from build123d import *

# Parameters (mm, degrees)
SKETCH1_R           = 1.0287
SKETCH1_R_2         = 1.47
BOSS_EXTRUDE1_DEPTH = 1.5875


with BuildPart() as part:
    # Sketch1 → Boss-Extrude1 (new body, symmetric)
    with BuildSketch(Plane.XY):
        Polygon((-12.5, 50), (-56.825, 50), (-56.825, 12.5), (-60, 12.5), (-60, -12.5), (-56.825, -12.5), (-56.825, -50), (-12.5, -50), (-12.5, -46.825), (-1.47, -46.825), (-1.47, -43.125), (-3.25, -43.125), (-3.25, -40.525), (-1.47, -40.525), (-1.47, -36.825), (1.47, -36.825), (1.47, -40.525), (3.25, -40.525), (3.25, -43.125), (1.47, -43.125), (1.47, -46.825), (12.5, -46.825), (12.5, -50), (56.825, -50), (56.825, -12.5), (60, -12.5), (60, 12.5), (56.825, 12.5), (56.825, 50), (12.5, 50), (12.5, 46.825), (1.47, 46.825), (1.47, 43.125), (3.25, 43.125), (3.25, 40.525), (1.47, 40.525), (1.47, 36.825), (-1.47, 36.825), (-1.47, 40.525), (-3.25, 40.525), (-3.25, 43.125), (-1.47, 43.125), (-1.47, 46.825), (-12.5, 46.825), align=None)
        with Locations((4.6, 2.575)):
            Circle(SKETCH1_R, mode=Mode.SUBTRACT)
        with Locations((25.4, 2.575)):
            Circle(SKETCH1_R, mode=Mode.SUBTRACT)
        with Locations((-58.4125, 0)):
            Circle(SKETCH1_R_2, mode=Mode.SUBTRACT)
        with Locations((58.4125, 0)):
            Circle(SKETCH1_R_2, mode=Mode.SUBTRACT)
    extrude(amount=BOSS_EXTRUDE1_DEPTH, both=True)


solid = part.part
The listing builds one solid part. Answer for the finished solid, in the listing's coordinates (mm). A direction names the side the tool comes from. Give positions to 0.01 mm unless a question says otherwise; leave off trailing zeros. Write each loop counter-clockwise with the first axis right and the second up, starting at its lowest first coordinate (ties: lowest second). Pieces come first, ordered by that corner, then holes. Notation, with made-up numbers: (-4, 79) - (54, 79) arc R27 cw to (54, 95) - close; hole circle Ø10 at (38, 88.5). An arc over 180 degrees is marked (long way). Use a Markdown table: item, result.
1. A tool of negligible diameter and unlimited length cuts with its end or side. For faces 1 (the flat face through (12.5, -48, 0)), 2 (the flat face through (-3.25, 42, 0)), 3 (the flat face through (-58, -12.5, 0)), 4 (the flat face through (-1.47, 45, 0)), from which of +Z, -Z, +X, -X, +Y, -Y can it reach the whole face along a straight path? Write none if from no direction.
Values follow:
| item | result |
|---|---|
| face 1 | +Z, -Z, -Y |
| face 2 | +Z, -Z |
| face 3 | +Z, -Z, -X, -Y |
| face 4 | +Z, -Z, +Y |
2. Find the intervals of material crossed by probe 1 along Y at (x, z) = (25.4, 0.7); probe 2 along Y at (x, z) = (0.5, 1.05) (3 decimals); probe 3 along X at (y, z) = (13.5, 1.35) (3 decimals), in increasing order. Write a range as from..to.
Values follow:
| item | result |
|---|---|
| probe 1 | y = -50..1.55, 3.6..50 |
| probe 2 | y = -36.825..36.825 |
| probe 3 | x = -56.825..56.825 |
3. Section A-A on y = 0 is taken. Write down the section's boundary in (x, z).
Values follow:
| item | result |
|---|---|
| outline | (-60, -1.59) - (-59.88, -1.59) - (-59.88, 1.59) - (-60, 1.59) - close; (-56.94, -1.59) - (56.94, -1.59) - (56.94, 1.59) - (-56.94, 1.59) - close; (59.88, -1.59) - (60, -1.59) - (60, 1.59) - (59.88, 1.59) - close |
4. Each of these flat-tipped pins is pushed along its axis until it touches: P1, Ø1.6, axis at y = 23.5, z = 0, coming from the -X side (3 decimals); P2, Ø0.5, axis at x = -2, z = 0, coming from the -Y side (3 decimals); P3, Ø1, axis at y = -38.5, z = 0.5, coming from the +X side (3 decimals). Where does it stop, or does it pass through?
Values follow:
| item | result |
|---|---|
| P1 | stops at x = -56.825 |
| P2 | stops at y = -46.825 |
| P3 | stops at x = 56.825 |
5. For a pull along X with two mould halves and no side action, classify faces 5 (the flat face through (-12.5, 48, 0)), 6 (the flat face through (-56.825, 32, 0)), 7 (the flat face through (34, -50, 0)) as released by +X, released by -X, zero draft, split by the parting line, or undercut.
Values follow:
| item | result |
|---|---|
| face 5 | undercut |
| face 6 | released by -X |
| face 7 | zero draft |
6. Section B-B on y = 22.5 is taken. Write down the section's boundary in (x, z) (1 decimal).
Values follow:
| item | result |
|---|---|
| outline | (-56.8, -1.6) - (56.8, -1.6) - (56.8, 1.6) - (-56.8, 1.6) - close |
7. Section C-C on z = -1 is taken. Count the separate pieces of the cut face and the enclosed holes in it, plus the area to 3 significant figures.
Values follow:
| item | result |
|---|---|
| separate pieces | 1 |
| enclosed holes | 4 |
| area | 11,300 mm² |
